Could you check a few things on this model? Use its own coordinates, in mm. A direction names the side the tool comes from. Coordinates: 2 decimals unless noted, no trailing zeros. Write each loop counter-clockwise with the first axis right and the second up, starting at its lowest first coordinate (ties: lowest second). Pieces come first, ordered by that corner, then holes.
```python
from build123d import *

# Parameters (mm, degrees)
F0_W     = 31.5
F0_H     = 48
F0_R     = 1.5
F0_R_2   = 14
F1_DEPTH = 1.2
F0_H_2   = 2
F2_DEPTH = 1.2
F3_DEPTH = 2.6
F4_DEPTH = 4


with BuildPart() as f1:
    # F0 (on Front) → F1 (new body)
    with BuildSketch(Plane.XZ):
        with Locations((0, -1)):
            Rectangle(F0_W, F0_H)
        with Locations((-10.75, -20)):
            Circle(F0_R, mode=Mode.SUBTRACT)
        with Locations((10.75, -20)):
            Circle(F0_R, mode=Mode.SUBTRACT)
        with Locations((0, -4)):
            Circle(F0_R_2, mode=Mode.SUBTRACT)
        with Locations((-10.75, 18)):
            Circle(F0_R, mode=Mode.SUBTRACT)
        with Locations((10.75, 18)):
            Circle(F0_R, mode=Mode.SUBTRACT)
    extrude(amount=F1_DEPTH)

    # F0 (on Front) → F2 (join)
    with BuildSketch(Plane.XZ):
        with Locations((0, 24)):
            Rectangle(F0_W, F0_H_2)
    extrude(amount=F2_DEPTH)

    # F0 (on Front) → F3 (join)
    with BuildSketch(Plane.XZ):
        with Locations((-10.75, 18)):
            Circle(F0_R)
        with Locations((10.75, 18)):
            Circle(F0_R)
        with Locations((10.75, -20)):
            Circle(F0_R)
        with Locations((-10.75, -20)):
            Circle(F0_R)
    extrude(amount=F3_DEPTH)

    # F0 (on Front) → F4 (join)
    with BuildSketch(Plane.XZ):
        with Locations((0, 24)):
            Rectangle(F0_W, F0_H_2)
    extrude(amount=F4_DEPTH)


solid = f1.part
```
Item 1: Which directions (+Z, -Z, +X, -X, +Y, -Y) give clear straight access to the entire face, cutting with the end or side of a thin tool? Please do faces 1 (the flat face through (11, -2.6, 18)), 2 (the flat face through (0, -4, 24)), 3 (the cylindrical face through (9.64, -1.89, 19.01)).
Item 2: I want a section at C-C, the plane z = -20. List the corners of the cut face in (x, y) for me, then the cut area to 3 significant figures.
Item 3: I want a section at A-A, the plane z = -4. List the corners of the cut face in (x, y) for me.
Item 4: If I drill on line 1 along Z through (x, y) = (0, -0.3); line 2 along Z through (x, y) = (7.5, -3.4); line 3 along Y through (x, z) = (13, 17.5), over which ranges is the centre line in solid material (lowest first)?
Item 5: Will these pins go through, and if not, where does the flat tip stop? pin 1 Ø1.5 at (x, z) = (11, -20) entering from -Y; pin 2 Ø2 at (x, y) = (-4, -2) entering from -Z; pin 3 Ø1.5 at (x, z) = (-3.5, 14) entering from -Y; pin 4 Ø2 at (x, y) = (0, -2.5) entering from -Z.
Item 6: If we mould it in two halves opening along X, with no side actions, what happens to faces 4 (the flat face through (-15.75, -1, 2)), 5 (the cylindrical face through (-11.86, -1.89, -18.99)), 6 (the flat face through (0, -3, 23))? For each: released by +X, released by -X, zero draft, split by the parting line, or undercut.
Item 7: I want a section at D-D, the plane x = -10. List the corners of the cut face in (y, z) for me.
Item 8: I want a section at B-B, the plane x = 0. List the corners of the cut face in (y, z) for me, then the cut area to 3 significant figures.
Taken from the geometry:
1. face 1: -Z, +X, -X, -Y
1. face 2: +Z, -Z, +X, -X, -Y
1. face 3: -Y
2. outline: (-15.75, -1.2) - (-12.25, -1.2) - (-12.25, -2.6) - (-9.25, -2.6) - (-9.25, -1.2) - (9.25, -1.2) - (9.25, -2.6) - (12.25, -2.6) - (12.25, -1.2) - (15.75, -1.2) - (15.75, 0) - (-15.75, 0) - close
2. area: 46.2 mm2
3. outline: (-15.75, -1.2) - (-14, -1.2) - (-14, 0) - (-15.75, 0) - close; (14, -1.2) - (15.75, -1.2) - (15.75, 0) - (14, 0) - close
4. line 1: z = -25 to -18, 10 to 25
4. line 2: z = 23 to 25
4. line 3: y = -1.2 to 0
5. pin 1: stops at y = -2.6
5. pin 2: stops at z = -25
5. pin 3: stops at y = -1.2
5. pin 4: stops at z = 23
6. face 4: released by -X
6. face 5: undercut
6. face 6: zero draft
7. outline: (-4, 23) - (-1.2, 23) - (-1.2, 19.3) - (-2.6, 19.3) - (-2.6, 16.7) - (-1.2, 16.7) - (-1.2, 5.8) - (0, 5.8) - (0, 25) - (-4, 25) - close; (-2.6, -21.3) - (-1.2, -21.3) - (-1.2, -25) - (0, -25) - (0, -13.8) - (-1.2, -13.8) - (-1.2, -18.7) - (-2.6, -18.7) - close
8. outline: (-4, 23) - (-1.2, 23) - (-1.2, 10) - (0, 10) - (0, 25) - (-4, 25) - close; (-1.2, -25) - (0, -25) - (0, -18) - (-1.2, -18) - close
8. area: 32.0 mm2
